from build123d import *

# Parameters (mm, degrees)
BASE_FLANGE1_DEPTH       = 574.9
EDGE_FLANGE1_DEPTH       = 767
M8_CLEARANCE_HOLE1_D     = 9
LPATTERN1_COUNT          = 6
LPATTERN1_PITCH          = 129
F_7_0_7_DIAMETER_HOLE1_D = 7
F_7_0_7_DIAMETER_HOLE2_D = 7
F_7_0_7_DIAMETER_HOLE3_D = 7
SKETCH17_W               = 286
SKETCH17_H               = 36
CUT_EXTRUDE1_DEPTH       = 2
M5_CLEARANCE_HOLE1_D     = 5.8
FILLET1_R                = 1


# Sheet-metal steps are written as plain solids
with BuildPart() as part:
    # Sketch1 → Base-Flange1 (new body)
    with BuildSketch(Plane(origin=(0, 0, 0), x_dir=(1, 0, 0), z_dir=(0, 1, 0))):
        with BuildLine():
            Line((25, 387.5), (4, 387.5))
            ThreePointArc((4, 387.5), (1.171572875, 386.328427125), (0, 383.5))
            Line((0, 383.5), (0, -383.5))
            ThreePointArc((0, -383.5), (1.171572875, -386.328427125), (4, -387.5))
            Line((4, -387.5), (25, -387.5))
            Line((25, -387.5), (25, -385.5))
            Line((25, -385.5), (4, -385.5))
            ThreePointArc((4, -385.5), (2.585786438, -384.914213562), (2, -383.5))
            Line((2, -383.5), (2, 383.5))
            ThreePointArc((2, 383.5), (2.585786438, 384.914213562), (4, 385.5))
            Line((4, 385.5), (25, 385.5))
            Line((25, 385.5), (25, 387.5))
        make_face()
    extrude(amount=BASE_FLANGE1_DEPTH)

    # Edge-Flange1 section (across the edge) → Edge-Flange1 (add)
    with BuildSketch(Plane(origin=(2, 576.9, -383.5), x_dir=(0, -1, 0), z_dir=(0, 0, 1))):
        with BuildLine():
            Line((-2, 2), (-2, 23))
            Line((-2, 23), (0, 23))
            Line((0, 23), (0, 2))
            ThreePointArc((0, 2), (0.585786438, 0.585786438), (2, 0))
            Line((2, 0), (2, -2))
            ThreePointArc((2, -2), (-0.828427125, -0.828427125), (-2, 2))
        make_face()
    extrude(amount=EDGE_FLANGE1_DEPTH)

    # M8 Clearance Hole1 (through all)
    with Locations(Plane(origin=(2, 0, 0), x_dir=(0, 0, -1), z_dir=(1, 0, 0))):
        with Locations((322.5, 15)):
            m8_clearance_hole1 = Hole(M8_CLEARANCE_HOLE1_D / 2)

    # LPattern1: M8 Clearance Hole1 ×6
    with Locations(*[(0, 0, i * LPATTERN1_PITCH) for i in range(1, LPATTERN1_COUNT)]):
        add(m8_clearance_hole1, mode=Mode.SUBTRACT)

    # Ø7.0 (7) Diameter Hole1 (through all)
    with Locations(Plane(origin=(0, 0, -387.5), x_dir=(-1, 0, 0), z_dir=(0, 0, -1))):
        with Locations((-16.5, 559.9), (-16.5, 469.083333333), (-16.5, 378.266666667), (-16.5, 287.45), (-16.5, 196.633333333), (-16.5, 105.816666667), (-16.5, 15)):
            Hole(F_7_0_7_DIAMETER_HOLE1_D / 2)

    # Ø7.0 (7) Diameter Hole2 (through all)
    with Locations(Plane(origin=(0, 576.9, 0), x_dir=(-1, 0, 0), z_dir=(0, -1, 0))):
        with Locations((-16.5, 363.5), (-16.5, 242.333333333), (-16.5, 121.166666667), (-16.5, 0), (-16.5, -121.166666667), (-16.5, -242.333333333), (-16.5, -363.5)):
            Hole(F_7_0_7_DIAMETER_HOLE2_D / 2)

    # Ø7.0 (7) Diameter Hole3 (through all)
    with Locations(Plane(origin=(0, 578.9, 0), x_dir=(1, 0, 0), z_dir=(0, 1, 0))):
        with Locations((16.5, -225), (16.5, -280)):
            Hole(F_7_0_7_DIAMETER_HOLE3_D / 2)

    # Sketch17 → Cut-Extrude1 (cut)
    with BuildSketch(Plane(origin=(2, 0, 0), x_dir=(0, 0, -1), z_dir=(1, 0, 0))):
        with Locations((0, 77)):
            Rectangle(SKETCH17_W, SKETCH17_H)
    extrude(amount=-CUT_EXTRUDE1_DEPTH, mode=Mode.SUBTRACT)

    # M5 Clearance Hole1 (through all)
    with Locations(Plane(origin=(2, 0, 0), x_dir=(0, 0, -1), z_dir=(1, 0, 0))):
        with Locations((-161, 77), (-161, 105), (-80.5, 105), (0, 105), (80.5, 105), (161, 105), (161, 77)):
            Hole(M5_CLEARANCE_HOLE1_D / 2)

    # Fillet1
    fillet1_edges = [part.edges().sort_by_distance(p)[0] for p in [
        (1, 59, 143),
        (1, 95, 143),
        (1, 95, -143),
        (1, 59, -143),
    ]]
    fillet(fillet1_edges, radius=FILLET1_R)


solid = part.part
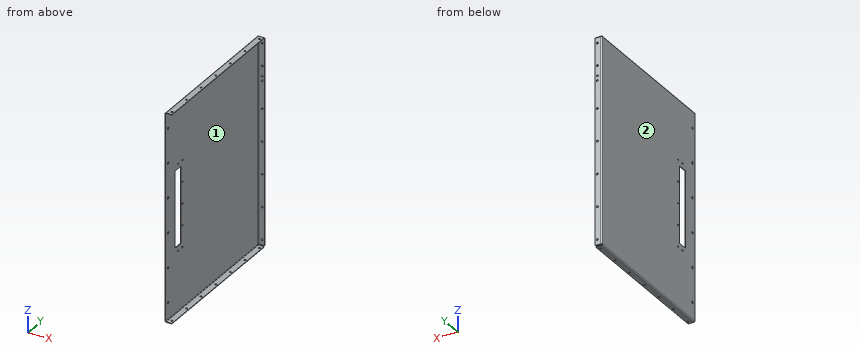
Part model, mm, in its own coordinate system. Face numbers are marked on the shaded views. Coordinates: 2 decimals unless noted, no trailing zeros. Write each loop counter-clockwise with the first axis right and the second up, starting at its lowest first coordinate (ties: lowest second). Pieces come first, ordered by that corner, then holes. Notation, with made-up numbers: (-18.5, 18.25) - (-10.5, 18.25) arc R27 cw to (-10.5, 57.25) - close; hole circle Ø5 at (-5, -14). An arc over 180 degrees is marked (long way). Put each result on its own line as item: value.
1. Band-saw the part on B-B (y = 332). Write the cut outline in (x, z).
Final values:
outline: (0, -383.5) arc R4 ccw to (4, -387.5) - (25, -387.5) - (25, -385.5) - (4, -385.5) arc R2 cw to (2, -383.5) - (2, 383.5) arc R2 cw to (4, 385.5) - (25, 385.5) - (25, 387.5) - (4, 387.5) arc R4 ccw to (0, 383.5) - close
2. Band-saw the part on C-C (z = 299). Write the cut outline in (x, y), then the cut area to 3 significant figures.
Final values:
outline: (0, 0) - (2, 0) - (2, 574.9) arc R2 cw to (4, 576.9) - (25, 576.9) - (25, 578.9) - (4, 578.9) arc R4 ccw to (0, 574.9) - close
area: 1,200 mm²
3. Flat gauge pins, fed straight in: pin 1 Ø1 at (x, z) = (22, -8) entering from -Y; pin 2 Ø2 at (x, z) = (13, -385) entering from +Y; pin 3 Ø1.5 at (y, z) = (338, -211.5) entering from +X. Where does each tip first touch, or does it go through?
Final values:
pin 1: stops at y = 576.9
pin 2: stops at y = 574.9
pin 3: stops at x = 2
4. Probe line 1 along Z through (x, y) = (15, 206); line 2 along Y through (x, z) = (23, -272); line 3 along Z through (x, y) = (2.5, 446.5). List the from-to ranges inside material, lowest first. Write a range as [from, to].
Final values:
line 1: z = [-387.5, -385.5], [385.5, 387.5]
line 2: y = [576.9, 578.9]
line 3: z = [-387.21, -384.82], [384.82, 387.21]
5. Band-saw the part on A-A (z = 13.5). Write the cut outline in (x, y), then the cut area to 3 significant figures.
Final values:
outline: (0, 0) - (2, 0) - (2, 59) - (0, 59) - close; (0, 95) - (2, 95) - (2, 574.9) arc R2 cw to (4, 576.9) - (25, 576.9) - (25, 578.9) - (4, 578.9) arc R4 ccw to (0, 574.9) - close
area: 1,130 mm²
6. Two-plate mould, pull along Z, no slides. Class the marked faces 1 and 2: +Z half, -Z half, draft (parallel to the pull), parting line (faces both ways), or undercut.
Final values:
face 1: undercut
face 2: draft
